from build123d import *

# Parameters (mm, degrees)
F0_W          = 38
F0_H          = 46
F2_DEPTH      = 10
F0_R          = 1.5
F3_DEPTH      = 0.6
F4_R          = 2
F5_DEPTH      = 25
F5_DEPTH_BACK = 25


with BuildPart() as f2:
    # F0 (on Front) → F2 (new body)
    with BuildSketch(Plane.XZ):
        Polygon((19, -47.5), (20, -47.5), (20, 47.5), (19, 47.5), (19, 44.5), (19, 0.5), (-19, 0.5), (-19, 47.5), (-20, 47.5), (-20, -47.5), align=None)
        with Locations((0, -23.5)):
            Rectangle(F0_W, F0_H, mode=Mode.SUBTRACT)
    extrude(amount=-F2_DEPTH)

    # F0 (on Front) → F3 (join)
    with BuildSketch(Plane.XZ):
        Polygon((19, 44.5), (19, 47.5), (-19, 47.5), (-19, 0.5), (19, 0.5), align=None)
        with Locations((-14, 44.5)):
            Circle(F0_R, mode=Mode.SUBTRACT)
        with Locations((14, 44.5)):
            Circle(F0_R, mode=Mode.SUBTRACT)
        with Locations((0, -23.5)):
            Rectangle(F0_W, F0_H)
    extrude(amount=-F3_DEPTH)

    # F4
    f4_edges = [f2.edges().sort_by_distance(p)[0] for p in [
        (-19, 0.6, 24),
        (0, 0.6, 0.5),
        (19, 0.6, 24),
        (-19, 0.6, -23.5),
        (0, 0.6, -0.5),
        (19, 0.6, -23.5),
        (0, 0.6, -46.5),
    ]]
    fillet(f4_edges, radius=F4_R)

    # F1 (on Right) → F5 (cut, two sides)
    with BuildSketch(Plane.YZ) as f5_sk:
        Polygon((10, -0.4571680084), (10, 31.2587800152), (10, 64.4635409117), (1, 64.4635409117), (0.6, 64.4635409117), (0.6, 29.3558231338), (1, 28.0871852128), (9.8558554806, 0), align=None)
    extrude(amount=-F5_DEPTH, mode=Mode.SUBTRACT)
    extrude(f5_sk.sketch, amount=F5_DEPTH_BACK, mode=Mode.SUBTRACT)


solid = f2.part
Read the model definition and answer for the solid it produces. Units are mm, in the model's axes. A direction names the side the tool comes from. Give positions to 0.01 mm unless a question says otherwise; leave off trailing zeros. Write each loop counter-clockwise with the first axis right and the second up, starting at its lowest first coordinate (ties: lowest second). Pieces come first, ordered by that corner, then holes. Notation, with made-up numbers: (4.5, 64) -> (9.5, 64) arc R15 cw to (9.5, 86) -> close; hole circle Ø2 at (33, 76.5). An arc over 180 degrees is marked (long way). Answer as a JSON object with one key per item and string values. Group by question number.
1) Find section C-C (x = -10). Write down the section's boundary in (y, z), and give its area (3 significant figures).
2) A tool of negligible diameter and unlimited length cuts with its end or side. For faces 5 (the cylindrical face through (13.675, 0.296, 43.036)), 6 (the flat face through (0, 6, -46.5)), 7 (the flat face through (-19, 5, 9)), from which of +Z, -Z, +X, -X, +Y, -Y can it reach the whole face along a straight path? Write none if from no direction.
3) Find section A-A (z = 44.5). Write down the section's boundary in (x, y).
4) Consider L1, parallel to X at y = 9.25, z = -28; L2, parallel to Z at x = 14, y = 0.1; L3, parallel to Z at x = 10, y = 6.25. Determine where each line is inside the solid, lowest interval first. Write a range as from..to.
5) Find section D-D (y = 6.5). Write down the section's boundary in (x, z), and give its area (3 significant figures).
6) Find section B-B (x = 14). Write down the section's boundary in (y, z), and give its area (3 significant figures).
7) The mould has two halves that part along Z. Classify faces 1 (the cylindrical face through (0.27, 1.2, 1.07)), 2 (the flat face through (0, 5, -47.5)), 3 (the cylindrical face through (18.4, 1.17, -23.18)), 4 (the flat face through (0, 10, -47)): +Z half, -Z half, draft (parallel to the pull), parting line (faces both ways), or undercut.
8) Each of these flat-tipped pins is pushed along its axis until it touches: P1, Ø3.5, axis at x = -6, y = 6.5, coming from the +Z side; P2, Ø1.5, axis at x = -4.5, z = -28, coming from the +Y side. Where does it stop, or does it pass through?
Values follow:
{
 "1": {"outline": "(0, -47.5) -> (10, -47.5) -> (10, -46.5) -> (2.6, -46.5) arc R2 cw to (0.6, -44.5) -> (0.6, -2.5) arc R2 cw to (2.6, -0.5) -> (10, -0.5) -> (10, -0.46) -> (9.7, 0.5) -> (2.6, 0.5) arc R2 cw to (0.6, 2.5) -> (0.6, 47.5) -> (0, 47.5) -> close", "area": "78.2 mm2"},
 "2": {"face 5": "+Y, -Y", "face 6": "+Y", "face 7": "+Z, +Y"},
 "3": {"outline": "(-20, 0) -> (-15.5, 0) -> (-15.5, 0.6) -> (-20, 0.6) -> close; (-12.5, 0) -> (12.5, 0) -> (12.5, 0.6) -> (-12.5, 0.6) -> close; (15.5, 0) -> (20, 0) -> (20, 0.6) -> (15.5, 0.6) -> close"},
 "4": {"L1": "x = -20..-19, 19..20", "L2": "z = -47.5..43, 46..47.5", "L3": "z = -47.5..-46.5, -0.5..0.5"},
 "5": {"outline": "(-20, -47.5) -> (20, -47.5) -> (20, 10.64) -> (19, 10.64) -> (19, 0.5) -> (-19, 0.5) -> (-19, 10.64) -> (-20, 10.64) -> close; hole (-19, -46.5) -> (19, -46.5) -> (19, -0.5) -> (-19, -0.5) -> close", "area": "192 mm2"},
 "6": {"outline": "(0, -47.5) -> (10, -47.5) -> (10, -46.5) -> (2.6, -46.5) arc R2 cw to (0.6, -44.5) -> (0.6, -2.5) arc R2 cw to (2.6, -0.5) -> (10, -0.5) -> (10, -0.46) -> (9.7, 0.5) -> (2.6, 0.5) arc R2 cw to (0.6, 2.5) -> (0.6, 43) -> (0, 43) -> close; (0, 46) -> (0.6, 46) -> (0.6, 47.5) -> (0, 47.5) -> close", "area": "76.4 mm2"},
 "7": {"face 1": "+Z half", "face 2": "-Z half", "face 3": "undercut", "face 4": "draft"},
 "8": {"P1": "stops at z = 0.5", "P2": "stops at y = 0.6"}
}
